Autodesk Inventor part; units mm, degrees
ref_plane "YZ Plane" through (0, 0, 0) normal (1, 0, 0) x (0, 1, 0)
ref_plane "XZ Plane" through (0, 0, 0) normal (0, 1, 0) x (-1, 0, 0)
ref_plane "XY Plane" through (0, 0, 0) normal (0, 0, 1) x (1, 0, 0)
sketch "Sketch1" plane through (0, 0, 0) normal (0, 0, 1) x (1, 0, 0)
  line L0 (-10.9402, 26.9819) -> (-10.9402, -11.1181)
  line L1 (-10.9402, -11.1181) -> (-9.6702, -11.1181)
  line L2 (-9.6702, -11.1181) -> (-9.6702, -7.9431)
  line L3 (-9.6702, -7.9431) -> (-4.8442, -7.9431)
  line L4 (-4.8442, -7.9431) -> (-4.8442, -6.6731)
  line L5 (-4.8442, -6.6731) -> (-9.6702, -6.6731)
  line L6 (-9.6702, -6.6731) -> (-9.6702, 22.5369)
  line L7 (-9.6702, 22.5369) -> (-4.8442, 22.5369)
  line L8 (-4.8442, 22.5369) -> (-4.8442, 23.8069)
  line L9 (-4.8442, 23.8069) -> (-9.6702, 23.8069)
  line L10 (-9.6702, 23.8069) -> (-9.6702, 26.9819)
  line L11 (-9.6702, 26.9819) -> (-10.9402, 26.9819)
  line L12 (-14.3692, 26.9819) -> (-14.3692, -11.1181) construction
  dimension "d0" = 9.525
  dimension "d1" = 4.699
  dimension "d2" = 38.1
  dimension "d3" = 3.175
  dimension "d4" = 1.27
  dimension "d5" = 1.27
revolve "Revolution1" add sketch "Sketch1" angle 360 about axis through (-14.3692, 26.9819, 0) along (0, -1, 0)
sketch "Sketch2" plane through (-14.3692, 23.8069, 0) normal (0, 1, 0) x (1, 0, 0)
  circle A0 centre (0, 0) radius 9.525
  point P0 (-5.715, 0)
  dimension "d18" = 5.715
hole "Hole1" at (-20.0842, 23.8069, 0) direction (0, -1, 0) diameter 1.5875 end up to surface
sketch "Sketch3" plane through (-14.3692, -7.9431, 0) normal (0, -1, 0) x (1, 0, 0)
  circle A0 centre (0, 0) radius 4.699
  line L0 (4.5878, 1.016) -> (5.715, 1.016)
  arc A1 (5.715, -1.016) -> (5.715, 1.016) centre (5.715, 0) ccw
  line L1 (5.715, -1.016) -> (4.5878, -1.016)
  dimension "d26" = 2.032
  dimension "d27" = 5.715
extrude "Extrusion1" add sketch "Sketch3" along normal up to surface (3.175 mm away) contours A0 L0 A1 L1
properties part number "bobbin" material "Delrin, Black"
Design review of the part built by this model. Coordinates are the model's own, in mm. A direction names the side the tool comes from. Coordinates: 2 decimals unless noted, no trailing zeros. Order: outer loops, then holes, each group sorted by start corner. A loop starts at its lowest first (then second) coordinate and runs counter-clockwise, first axis right, second up.
1) Take a section at A-A, the plane z = -7. Give the boundary of the cut face in (x, y), and give its area (3 significant figures).
2) Mouldability with a two-part tool opening along Z and no side actions: class faces 1 (the cylindrical face through (-21.928, -7.299, 5.796)), 2 (the cylindrical face through (-11.2, 7.67, -1.31)), 3 (the flat face through (-19, -6.673, -2)) as +Z half, -Z half, draft (parallel to the pull), parting line (faces both ways), or undercut.
3) Wall thickness on line 1 along Z through (x, y) = (-14.25, 11.5); line 2 along Y through (x, z) = (-21.75, 3.75); line 3 along X through (y, z) = (-3, -0.5): over which ranges is each line inside the solid? List them lowest first.
4) For faces 4 (the cylindrical face through (-9.887, 25.417, -1.411)), 5 (the flat face through (-19, -7.943, -2)), 6 (the cylindrical face through (-7.64, -9.51, 0.02)), 7 (the flat face through (-9, -10, 1.016)), 8 (the cylindrical face through (-9.887, 8.136, -1.411)), list the 3-axis set-ups (+Z, -Z, +X, -X, +Y, -Y) from which the entire face can be reached by the end or side of a thin tool; tool diameter is ignored.
5) Take a section at D-D, the plane x = -11.5. Give the boundary of the cut face in (y, z), and give its area (3 significant figures).
6) Clearance check with flat-ended pins moving along their axes: pin 1 (9.5 mm diameter, centred on x = -13, z = 2.5, fed in from +Y); pin 2 (3 mm diameter, centred on y = 3.5, z = -1.5, fed in from -X); pin 3 (5 mm diameter, centred on x = -20.5, y = 18, fed in from +Z); pin 4 (6 mm diameter, centred on x = -10.5, z = -7, fed in from -Y). State where each tip first meets the part, or that it passes through.
7) Take a section at B-B, the plane z = 0. Give the boundary of the cut face in (x, y).
8) Take a section at C-C, the plane y = 7.5. Give the boundary of the cut face in (x, z).
Returned:
1. outline: (-20.83, -7.94) - (-7.91, -7.94) - (-7.91, -6.67) - (-20.83, -6.67) - close; (-20.83, 22.54) - (-7.91, 22.54) - (-7.91, 23.81) - (-20.83, 23.81) - close
1. area: 32.8 mm2
2. face 1: parting line
2. face 2: undercut
2. face 3: draft
3. line 1: z = -4.7 to -3.43, 3.43 to 4.7
3. line 2: y = -7.94 to -6.67, 22.54 to 23.81
3. line 3: x = -19.04 to -17.76, -10.98 to -9.7
4. face 4: +Y
4. face 5: -Y
4. face 6: +X, -Y
4. face 7: +Z, +X, -Y
4. face 8: none
5. outline: (-11.12, -3.72) - (-7.94, -3.72) - (-7.94, -9.08) - (-6.67, -9.08) - (-6.67, -3.72) - (22.54, -3.72) - (22.54, -9.08) - (23.81, -9.08) - (23.81, -3.72) - (26.98, -3.72) - (26.98, -1.88) - (-11.12, -1.88) - close; (-11.12, 1.88) - (26.98, 1.88) - (26.98, 3.72) - (23.81, 3.72) - (23.81, 9.08) - (22.54, 9.08) - (22.54, 3.72) - (-6.67, 3.72) - (-6.67, 9.08) - (-7.94, 9.08) - (-7.94, 3.72) - (-11.12, 3.72) - close
5. area: 168 mm2
6. pin 1: stops at y = 26.98
6. pin 2: stops at x = -19.07
6. pin 3: stops at z = 2.98
6. pin 4: stops at y = -7.94
7. outline: (-23.89, -7.94) - (-19.07, -7.94) - (-19.07, -11.12) - (-17.8, -11.12) - (-17.8, 26.98) - (-19.07, 26.98) - (-19.07, 23.81) - (-19.29, 23.81) - (-19.29, 22.54) - (-19.07, 22.54) - (-19.07, -6.67) - (-23.89, -6.67) - close; (-23.89, 22.54) - (-20.88, 22.54) - (-20.88, 23.81) - (-23.89, 23.81) - close; (-10.94, -11.12) - (-7.64, -11.12) - (-7.64, -7.94) - (-4.84, -7.94) - (-4.84, -6.67) - (-9.67, -6.67) - (-9.67, 22.54) - (-4.84, 22.54) - (-4.84, 23.81) - (-9.67, 23.81) - (-9.67, 26.98) - (-10.94, 26.98) - close
8. outline: circle Ø9.4 at (-14.37, 0); hole circle Ø6.86 at (-14.37, 0)
